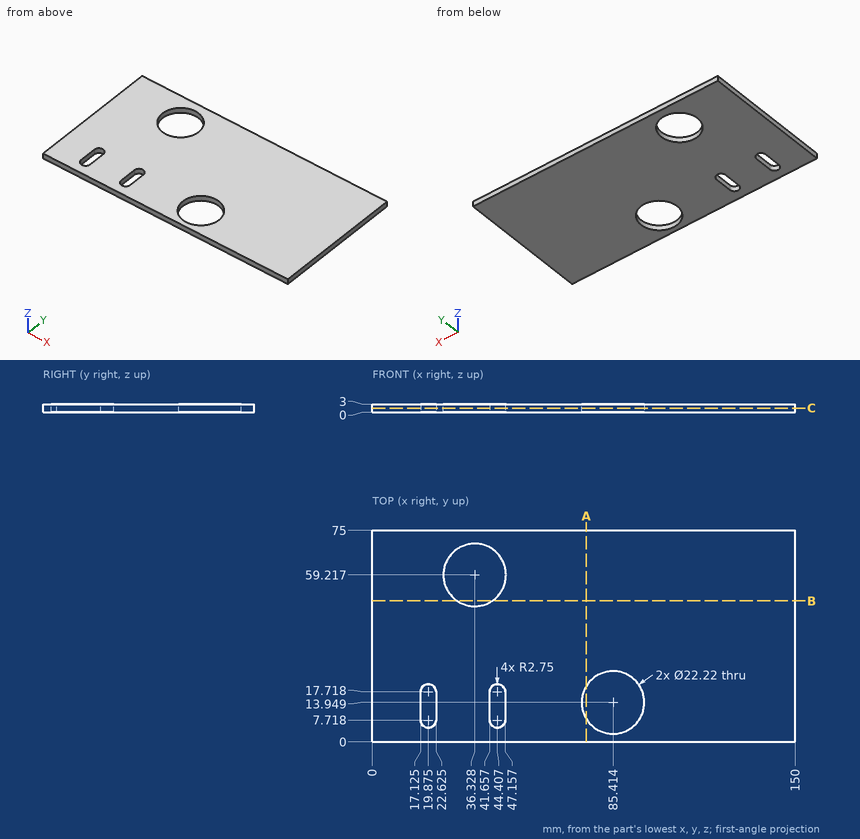
Can you work these out from the drawing? Everything is in mm from the part's minimum corner. Give positions to 0.01 mm unless a question says otherwise; leave off trailing zeros. Write each loop counter-clockwise with the first axis right and the second up, starting at its lowest first coordinate (ties: lowest second). Pieces come first, ordered by that corner, then holes. Notation, with made-up numbers: (8.5, -39.75) -> (17.5, -39.75) arc R25 ccw to (17.5, -14.75) -> close; hole circle Ø9 at (55, -8). An arc over 180 degrees is marked (long way). Write each question's results on one line, items separated by ' | '.
Item 1: Suppose I cut it at A-A on x = 76. Write out the boundary of the cut face in (y, z).
Output:
outline: (0, 0) -> (8.05, 0) -> (8.05, 3) -> (0, 3) -> close; (19.85, 0) -> (75, 0) -> (75, 3) -> (19.85, 3) -> close
Item 2: If I drill on L1, parallel to Y at x = 44, z = 0.55 (1 decimal); L2, parallel to X at y = 6.5, z = 1.05 (1 decimal); L3, parallel to Y at x = 30.5, z = 0.9 (1 decimal), over which ranges is the centre line in solid material (lowest first)?
Output:
L1: y = 0 to 5, 20.4 to 51.2, 67.3 to 75 | L2: x = 0 to 17.4, 22.3 to 41.9, 46.9 to 77.2, 93.7 to 150 | L3: y = 0 to 49.8, 68.7 to 75
Item 3: Suppose I cut it at C-C on z = 1.55. Give the number of separate pieces and of enclosed holes in the cut face, plus the area to 3 significant figures.
Output:
separate pieces: 1 | enclosed holes: 4 | area: 10,300 mm^2
Item 4: Suppose I cut it at B-B on y = 50. Write out the boundary of the cut face in (x, z) (1 decimal), plus the area to 3 significant figures.
Output:
outline: (0, 0) -> (30.1, 0) -> (30.1, 3) -> (0, 3) -> close; (42.5, 0) -> (150, 0) -> (150, 3) -> (42.5, 3) -> close | area: 413 mm^2
